from build123d import *

# Parameters (mm, degrees)
F2_R     = 5
F3_DEPTH = 25


with BuildPart() as f1:
    # F0 (on Front) → F1 (revolve)
    with BuildSketch(Plane.XZ):
        Polygon((-30, 50), (-57.5, 50), (-57.5, 45), (-35, 45), (-35, -5), (0, -5), (0, 0), (-30, 0), align=None)
    revolve(axis=Axis((0, 0, 20.000002), (0, 0, -1)))

    # F2 (on face) → F3 (cut)
    with BuildSketch(Plane.XY.offset(50)):
        with Locations((0, 45)):
            Circle(F2_R)
        with Locations((-45, 0)):
            Circle(F2_R)
        with Locations((0, -45)):
            Circle(F2_R)
        with Locations((45, 0)):
            Circle(F2_R)
    extrude(amount=-F3_DEPTH, mode=Mode.SUBTRACT)


solid = f1.part
Work out the finished part from the listing and answer in its coordinate system (mm). A direction names the side the tool comes from. Coordinates: 2 decimals unless noted, no trailing zeros. Write each loop counter-clockwise with the first axis right and the second up, starting at its lowest first coordinate (ties: lowest second). Pieces come first, ordered by that corner, then holes. Notation, with made-up numbers: M -12,-25.5 L 1,-25.5 A21 ccw 1,6.5 Z; hole C 54.25,-32 d10. An arc over 180 degrees is marked long. Write item = value, one per line.
1. Flat-ended cylindrical pins translate along their axes: pin 1 (10 mm diameter, centred on x = -30.5, y = -27, fed in from -Z); pin 2 (6 mm diameter, centred on x = 45, y = 0, fed in from -Z); pin 3 (1 mm diameter, centred on x = -23.5, z = 27, fed in from +Y); pin 4 (5 mm diameter, centred on y = -34.5, z = 25.5, fed in from -X). Find the tip coordinate at first contact, or state that the pin passes through.
Solution:
pin_1 = 45
pin_2 = through
pin_3 = 26.38
pin_4 = -14.18
2. For faces 4 (the face through (29.97, 1.32, 25.35)), 5 (the face through (12.465, -56.133, 47.465)), determine the directions among +Z, -Z, +X, -X, +Y, -Y from which every point of the face is accessible in a straight line to the end or side of a thin tool.
Solution:
face_4 = +Z
face_5 = +Z, -Z
3. Determine the mould class of faces 1 (the face through (40, 0, 48)), 2 (the face through (28, -21, 20)), 3 (the face through (-25, -25, 45)) for opening direction X: released by +X, released by -X, zero draft, split by the parting line, or undercut.
Solution:
face_1 = undercut
face_2 = split by the parting line
face_3 = zero draft
4. Straight lines are drawn through the part: line 1 (Y direction, x = 0, z = 48); line 2 (Y direction, x = 0, z = 16); line 3 (Z direction, x = -24, y = 49.5). For each, find the intervals that lie inside material, in ascending order. Write a range as from..to.
Solution:
line_1 = -57.5..-50, -40..-30, 30..40, 50..57.5
line_2 = -35..-30, 30..35
line_3 = 45..50
5. The part is cut by section D-D (x = -48.5). Determine the outline of the cut face in (y, z).
Solution:
outline = M -30.89,45 L -3.57,45 L -3.57,50 L -30.89,50 Z; M 3.57,45 L 30.89,45 L 30.89,50 L 3.57,50 Z
6. The part is cut by section A-A (x = -0.5). Determine the outline of the cut face in (y, z), then the cut area to 3 significant figures.
Solution:
outline = M -57.5,45 L -49.97,45 L -49.97,50 L -57.5,50 Z; M -40.03,45 L -35,45 L -35,-5 L 35,-5 L 35,45 L 40.03,45 L 40.03,50 L 30,50 L 30,0 L -30,0 L -30,50 L -40.03,50 Z; M 49.97,45 L 57.5,45 L 57.5,50 L 49.97,50 Z
area = 976 mm2
7. The part is cut by section C-C (z = 46.5). Determine the outline of the cut face in (x, y).
Solution:
outline = C 0,0 d115; hole C -45,0 d10; hole C 0,0 d60; hole C 0,-45 d10; hole C 0,45 d10; hole C 45,0 d10
8. The part is cut by section B-B (y = -45). Determine the outline of the cut face in (x, z).
Solution:
outline = M -35.79,45 L -5,45 L -5,50 L -35.79,50 Z; M 5,45 L 35.79,45 L 35.79,50 L 5,50 Z
